from build123d import *

# Parameters (mm, degrees)
CYLINDER_R           = 2.15
CYLINDER_DEPTH       = 50
CYLINDER_PITCH_ANGLE = 90
BOX002_W             = 14
BOX002_H             = 11
BOX002_DEPTH         = 20.5
CHAMFER_SIZE         = 4
FILLET001_R          = 5
BOX003_W             = 14
BOX003_H             = 25
BOX003_DEPTH         = 4
BOX003_ROLL_ANGLE    = -15
BOX004_W             = 14
BOX004_H             = 2.5
BOX004_DEPTH         = 5
POCKET006_DEPTH      = 15
SKETCH008_W          = 0.2
SKETCH008_H          = 34.34452
POCKET008_DEPTH      = 80


with BuildPart() as cylinder:
    # Cylinder → Cylinder (new body)
    with BuildSketch(Plane.XY):
        Circle(CYLINDER_R)
    extrude(amount=CYLINDER_DEPTH)


with BuildPart() as cylinder_1:
    # Cylinder pitch: moved
    add(cylinder.part.rotate(Axis((0, 0, 0), (0, 1, 0)), CYLINDER_PITCH_ANGLE))


with BuildPart() as cylinder_2:
    # Cylinder placement: moved
    add(cylinder_1.part.moved(Location((31, -6, 12.9))))


with BuildPart() as fillet001:
    # Box002 → Box002 (new body)
    with BuildSketch(Plane(origin=(52, -12, -3), x_dir=(1, 0, 0), z_dir=(0, 0, 1))):
        with Locations((7, 5.5)):
            Rectangle(BOX002_W, BOX002_H)
    extrude(amount=BOX002_DEPTH)

    # Chamfer
    chamfer_edges = [fillet001.edges().sort_by_distance(p)[0] for p in [
        (59, -1, -3),
    ]]
    chamfer(chamfer_edges, length=CHAMFER_SIZE)

    # Fillet001
    fillet001_edges = [fillet001.edges().sort_by_distance(p)[0] for p in [
        (59, -1, 17.5),
    ]]
    fillet(fillet001_edges, radius=FILLET001_R)


with BuildPart() as cube002:
    # Box003 → Box003 (new body)
    with BuildSketch(Plane.XY):
        with Locations((7, 12.5)):
            Rectangle(BOX003_W, BOX003_H)
    extrude(amount=BOX003_DEPTH)


with BuildPart() as cube002_1:
    # Box003 roll: moved
    add(cube002.part.rotate(Axis((0, 0, 0), (1, 0, 0)), BOX003_ROLL_ANGLE))


with BuildPart() as cube002_2:
    # Box003 placement: moved
    add(cube002_1.part.moved(Location((52, -12, -3))))


with BuildPart() as pocket008:
    # Box004 → Box004 (new body)
    with BuildSketch(Plane(origin=(52, -12, 14), x_dir=(1, 0, 0), z_dir=(0, 0, 1))):
        with Locations((7, 1.25)):
            Rectangle(BOX004_W, BOX004_H)
    extrude(amount=BOX004_DEPTH)

    # Fusion: union Fillet001, Cube002
    add(fillet001.part)
    add(cube002_2.part)

    # Cut001: cut Cylinder
    add(cylinder_2.part, mode=Mode.SUBTRACT)

    # Sketch006 → Pocket006 (cut)
    with BuildSketch(Plane.YZ.offset(66)):
        Polygon((13.183422, -5.606773), (-4.041064, -0.991486), (-0.407217, 12.570217), align=None)
    extrude(amount=-POCKET006_DEPTH, mode=Mode.SUBTRACT)

    # Sketch008 → Pocket008 (cut)
    with BuildSketch(Plane.XZ.offset(12)):
        with Locations((52.1, 9.746044)):
            Rectangle(SKETCH008_W, SKETCH008_H)
    extrude(amount=-POCKET008_DEPTH, mode=Mode.SUBTRACT)


solid = pocket008.part
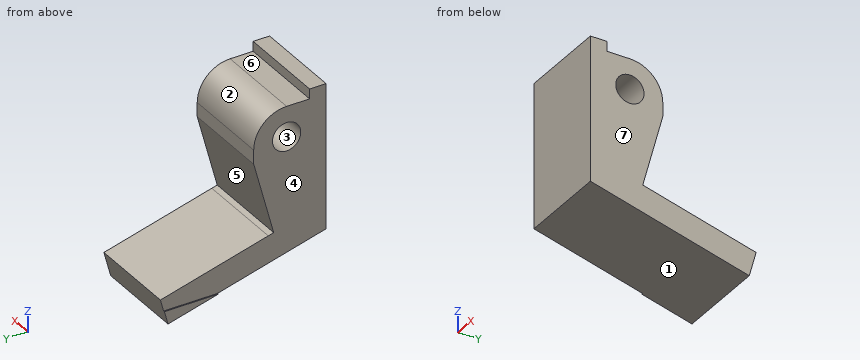
Here's how the part is built. I have some questions about the finished solid (model axes, mm). Face numbers are marked on the shaded views. A direction names the side the tool comes from. Give positions to 0.01 mm unless a question says otherwise; leave off trailing zeros. Order: outer loops, then holes, each group sorted by start corner. A loop starts at its lowest first (then second) coordinate and runs counter-clockwise, first axis right, second up. Notation, with made-up numbers: (-19, 62) -> (-6, 62) arc R18 ccw to (-6, 88) -> close; hole circle Ø7 at (-3, 46.25). An arc over 180 degrees is marked (long way). One line per item, written item: value. Start each with the question number.
1. I need wall thicknesses on probe 1 along X at (y, z) = (-8, 10.5); probe 2 along Y at (x, z) = (55.75, 12.9); probe 3 along Z at (x, y) = (57.25, -6.75). Which ranges of each line are inside material? Lowest first, please. Write a range as from..to.
2. Imagine slicing it at B-B, the plane z = 14. List the corners of the cut face in (x, y) for me.
3. We'd pull the mould along Z, two halves only. Please class the marked faces 1, 2, 3 and 4: released by +Z, released by -Z, zero draft, split by the parting line, or undercut.
4. Imagine slicing it at D-D, the plane y = 7.75. List the corners of the cut face in (x, z) for me.
5. Imagine slicing it at C-C, the plane y = -1.5. List the corners of the cut face in (x, z) for me.
6. Will these pins go through, and if not, where does the flat tip stop? pin 1 Ø5 at (x, z) = (59.5, 15.5) entering from +Y; pin 2 Ø4 at (y, z) = (-6, 12.9) entering from -X.
7. Imagine slicing it at A-A, the plane x = 63.25. List the corners of the cut face in (y, z) for me.
8. For the marked faces 5, 6 and 7, which set-ups out of +Z, -Z, +X, -X, +Y, -Y let a thin tool reach every point of the face, with its end or its side?
Values follow:
1. probe 1: x = 52.2..66
1. probe 2: y = -12..-8.15, -3.85..-1.02
1. probe 3: z = -4.41..10.89, 14.91..17.5
2. outline: (52.2, -12) -> (66, -12) -> (66, -7.85) -> (52.2, -7.85) -> close; (52.2, -4.15) -> (66, -4.15) -> (66, -1.23) -> (52.2, -1.23) -> close
3. face 1: released by -Z
3. face 2: released by +Z
3. face 3: undercut
3. face 4: zero draft
4. outline: (52, -8.29) -> (66, -8.29) -> (66, -4.15) -> (52.2, -4.15) -> (52.2, -7.43) -> (52, -7.43) -> close
5. outline: (52.2, -5.81) -> (66, -5.81) -> (66, -1.67) -> (52.2, -1.67) -> close; (52.2, 8.49) -> (66, 8.49) -> (66, 14.68) -> (52.2, 14.68) -> close
6. pin 1: stops at y = -1.03
6. pin 2: passes through
7. outline: (-12, -3) -> (12.15, -9.47) -> (13.18, -5.61) -> (-4.04, -0.99) -> (-1, 10.36) -> (-1, 12.5) arc R5 ccw to (-6, 17.5) -> (-9.5, 17.5) -> (-9.5, 19) -> (-12, 19) -> close; hole circle Ø4.3 at (-6, 12.9)
8. face 5: +X, -X, +Y
8. face 6: +Z, +X, -X, +Y
8. face 7: +Z, -Z, +X, +Y, -Y
